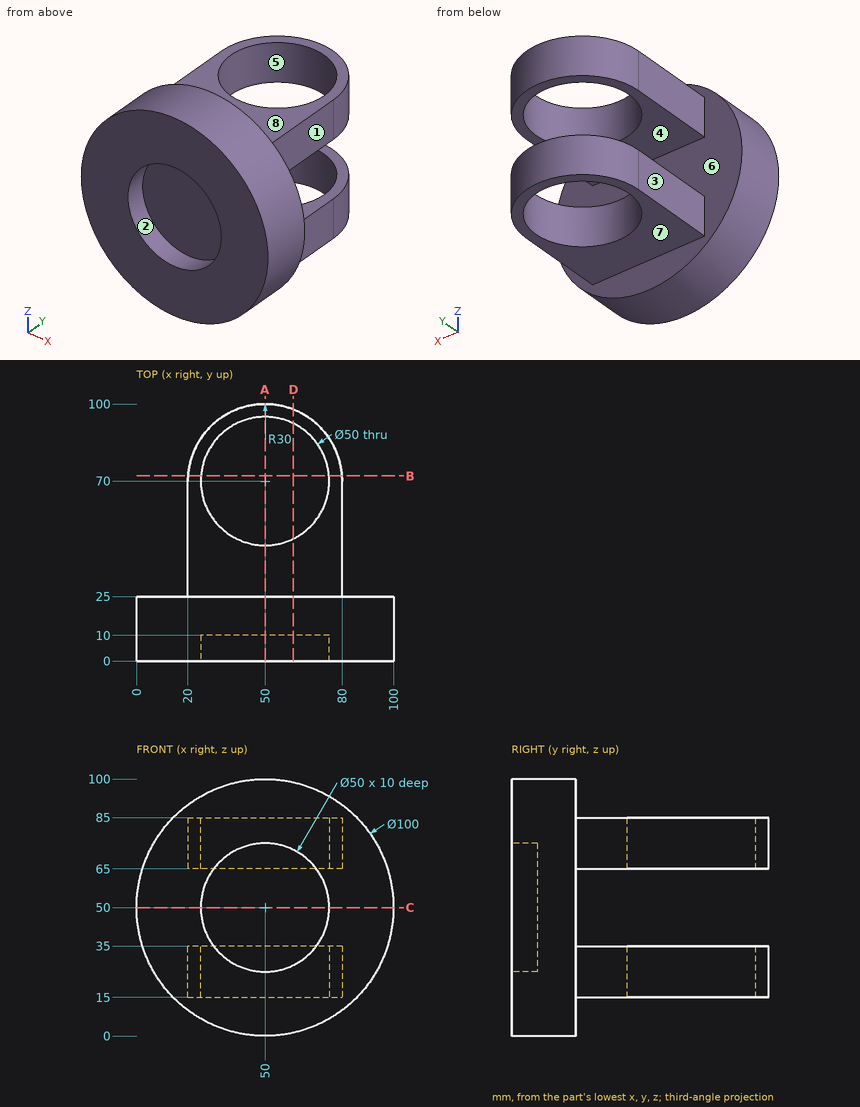
Design review of the part shown in the three views and the two pictorial views. Dimensions are in mm from the part's minimum x, y and z. A direction names the side the tool comes from. Round coordinates to 2 decimals unless told otherwise and drop trailing zeros. Write each loop counter-clockwise with the first axis right and the second up, starting at its lowest first coordinate (ties: lowest second). Pieces come first, ordered by that corner, then holes.
Item 1: We need section D-D on x = 61. Write out the cut boundary in (y, z) (3 decimals), and give its area (3 significant figures).
Item 2: Clearance check with flat-ended pins moving along their axes: pin 1 Ø3 at (y, z) = (21.5, 43.5) entering from +X; pin 2 Ø4 at (y, z) = (72.5, 14) entering from -X; pin 3 Ø22 at (y, z) = (50.5, 73.5) entering from +X. State where each tip first meets the part, or that it passes through.
Item 3: The part is to be moulded in two halves that separate along Z. For the marked faces 5, 6, 7 and 8, say which applies: +Z half, -Z half, draft (parallel to the pull), parting line (faces both ways), or undercut.
Item 4: For the marked faces 1, 2, 3 and 4, list the 3-axis set-ups (+Z, -Z, +X, -X, +Y, -Y) from which the entire face can be reached by the end or side of a thin tool; tool diameter is ignored.
Item 5: We need section B-B on y = 72. Write out the cut boundary in (x, z).
Item 6: For probe 1 along X at (y, z) = (70.5, 68.5) (3 decimals); probe 2 along Z at (x, y) = (50, 7.5); probe 3 along Y at (x, z) = (50, 80), list the stretches that pass through material, from the lowest coordinate up.
Item 7: We need section C-C on z = 50. Write out the cut boundary in (x, y).
Item 8: We need section A-A on x = 50. Write out the cut boundary in (y, z), and give its area (3 significant figures).
Returned:
1. outline: (0, 1.225) - (25, 1.225) - (25, 15) - (47.55, 15) - (47.55, 35) - (25, 35) - (25, 65) - (47.55, 65) - (47.55, 85) - (25, 85) - (25, 98.775) - (0, 98.775) - (0, 72.45) - (10, 72.45) - (10, 27.55) - (0, 27.55) - close; (92.45, 15) - (97.911, 15) - (97.911, 35) - (92.45, 35) - close; (92.45, 65) - (97.911, 65) - (97.911, 85) - (92.45, 85) - close
1. area: 3,110 mm2
2. pin 1: stops at x = 99.75
2. pin 2: stops at x = 20.01
2. pin 3: stops at x = 80
3. face 5: draft
3. face 6: undercut
3. face 7: -Z half
3. face 8: +Z half
4. face 1: +Z, -Z, +X, +Y
4. face 2: -Y
4. face 3: +Z, -Z, -X, +Y
4. face 4: +X, -X, +Y
5. outline: (20.07, 15) - (25.08, 15) - (25.08, 35) - (20.07, 35) - close; (20.07, 65) - (25.08, 65) - (25.08, 85) - (20.07, 85) - close; (74.92, 15) - (79.93, 15) - (79.93, 35) - (74.92, 35) - close; (74.92, 65) - (79.93, 65) - (79.93, 85) - (74.92, 85) - close
6. probe 1: x = 20.004 to 25.005, 74.995 to 79.996
6. probe 2: z = 0 to 25, 75 to 100
6. probe 3: y = 0 to 45, 95 to 100
7. outline: (0, 0) - (25, 0) - (25, 10) - (75, 10) - (75, 0) - (100, 0) - (100, 25) - (0, 25) - close
8. outline: (0, 0) - (25, 0) - (25, 15) - (45, 15) - (45, 35) - (25, 35) - (25, 65) - (45, 65) - (45, 85) - (25, 85) - (25, 100) - (0, 100) - (0, 75) - (10, 75) - (10, 25) - (0, 25) - close; (95, 15) - (100, 15) - (100, 35) - (95, 35) - close; (95, 65) - (100, 65) - (100, 85) - (95, 85) - close
8. area: 3,000 mm2
